from build123d import *

# Parameters (mm, degrees)
F1_DEPTH = 22.5
F2_DEPTH = 25
F3_R     = 5
F5_D     = 22
F5_DEPTH = 6
F5_TIP   = 6.6094668093
F6_D     = 22
F6_DEPTH = 6
F6_TIP   = 6.6094668093
F8_D     = 22
F8_DEPTH = 6
F8_TIP   = 6.6094668093
F9_D     = 22
F9_DEPTH = 6
F9_TIP   = 6.6094668093


with BuildPart() as f1:
    # F0 (on Right) → F1 (new body, symmetric)
    with BuildSketch(Plane.YZ):
        with BuildLine():
            Line((-50, -20), (50, -20))
            Line((50, -20), (37.9778109491, -11.483842507))
            add(Edge.make_bspline(
                [(37.9778109491, -11.483842507), (33.7362140417, -8.5331639275), (28.4293044028, -5.4691263704), (19.5910925664, -4.9491255013), (14.8890013853, -4.8763493822)],
                knots=[0, 0, 0, 0, 0.441705983, 0.8114966727, 0.8114966727, 0.8114966727, 0.8114966727], degree=3))
            Line((14.8890013853, -4.8763493822), (-3.1495152507, 6.404644344))
            Line((-3.1495152507, 6.404644344), (-25.2773519605, 6.404644344))
            Line((-25.2773519605, 6.404644344), (-32.455407083, -4.2915642262))
            Line((-32.455407083, -4.2915642262), (-50, -4.2915642262))
            Line((-50, -4.2915642262), (-50, -20))
        make_face()
    extrude(amount=F1_DEPTH, both=True)

    # F0 (on Right) → F2 (join)
    with BuildSketch(Plane.YZ):
        with BuildLine():
            Line((-50, -20), (50, -20))
            Line((50, -20), (37.9778109491, -11.483842507))
            add(Edge.make_bspline(
                [(37.9778109491, -11.483842507), (33.7362140417, -8.5331639275), (28.4293044028, -5.4691263704), (19.5910925664, -4.9491255013), (14.8890013853, -4.8763493822)],
                knots=[0, 0, 0, 0, 0.441705983, 0.8114966727, 0.8114966727, 0.8114966727, 0.8114966727], degree=3))
            Line((14.8890013853, -4.8763493822), (-3.1495152507, 6.404644344))
            Line((-3.1495152507, 6.404644344), (-25.2773519605, 6.404644344))
            Line((-25.2773519605, 6.404644344), (-32.455407083, -4.2915642262))
            Line((-32.455407083, -4.2915642262), (-50, -4.2915642262))
            Line((-50, -4.2915642262), (-50, -20))
        make_face()
    extrude(amount=F2_DEPTH)

    # F3
    f3_edges = [f1.edges().sort_by_distance(p)[0] for p in [
        (1.25, -25.277352, 6.404644),
        (1.25, -32.455407, -4.291564),
        (1.25, -50, -4.291564),
        (1.25, -3.149515, 6.404644),
        (-11.25, 14.889001, -4.876349),
        (23.75, 14.889001, -4.876349),
        (11.25, 14.889001, -4.876349),
    ]]
    fillet(f3_edges, radius=F3_R)

    # F5
    with Locations(Plane.YZ.offset(25)):
        with Locations((-31.3936918974, -20)):
            Hole(F5_D / 2, depth=F5_DEPTH)
            with Locations((0, 0, -(F5_DEPTH + F5_TIP / 2))):  # 118° drill point
                Cone(0, F5_D / 2, F5_TIP, mode=Mode.SUBTRACT)

    # F6
    with Locations(Plane.YZ.offset(25)):
        with Locations((19.693158567, -20)):
            Hole(F6_D / 2, depth=F6_DEPTH)
            with Locations((0, 0, -(F6_DEPTH + F6_TIP / 2))):  # 118° drill point
                Cone(0, F6_D / 2, F6_TIP, mode=Mode.SUBTRACT)

    # F8
    with Locations(Plane(origin=(-22.5, 0, 0), x_dir=(0, -1, 0), z_dir=(-1, 0, 0))):
        with Locations((-19.701551646, -20)):
            Hole(F8_D / 2, depth=F8_DEPTH)
            with Locations((0, 0, -(F8_DEPTH + F8_TIP / 2))):  # 118° drill point
                Cone(0, F8_D / 2, F8_TIP, mode=Mode.SUBTRACT)

    # F9
    with Locations(Plane(origin=(-22.5, 0, 0), x_dir=(0, -1, 0), z_dir=(-1, 0, 0))):
        with Locations((31.4156152308, -20)):
            Hole(F9_D / 2, depth=F9_DEPTH)
            with Locations((0, 0, -(F9_DEPTH + F9_TIP / 2))):  # 118° drill point
                Cone(0, F9_D / 2, F9_TIP, mode=Mode.SUBTRACT)


solid = f1.part
Design review of the part built by this model. Coordinates are the model's own, in mm. A direction names the side the tool comes from. Round coordinates to 2 decimals unless told otherwise and drop trailing zeros. Order: outer loops, then holes, each group sorted by start corner. A loop starts at its lowest first (then second) coordinate and runs counter-clockwise, first axis right, second up. Notation, with made-up numbers: M 38.5,17.5 L 77.5,17.5 A15 cw 77.5,27.5 Z; hole C 63,81.25 d3. An arc over 180 degrees is marked long. Answer as CSV lines item,"result". Start each with the question number.
1) For pin 1 Ø4 at (y, z) = (20.5, -5) entering from +X; pin 2 Ø2 at (x, z) = (9, -14) entering from +Y; pin 3 Ø4 at (y, z) = (15, -2.5) entering from +X (3 decimals); pin 4 Ø1.5 at (x, z) = (-15, -6.5) entering from +Y, all flat-tipped, find the tip position at first contact; note any pin that passes through.
2) Tool access review of faces 1 (the face through (1, -40, -4.292)), 2 (the face through (1, -50, -15)), 3 (the face through (22, 19.5, -9)): name each direction out of +Z, -Z, +X, -X, +Y, -Y from which nothing blocks a thin tool from reaching the whole face with its end or side.
3) Add section B-B (y = 0). Give the boundary of the cut face in (x, z).
4) Add section A-A (z = 2). Give the boundary of the cut face in (x, y), then the cut area to 3 significant figures.
5) Wall thickness on line 1 along Y through (x, z) = (-13, -16.75); line 2 along Y through (x, z) = (17, -17); line 3 along Z through (x, y) = (-1.5, -35): over which ranges is each line inside the solid? List them lowest first. Write a range as [from, to].
6) The part is to be moulded in two halves that separate along Y. For faces 4 (the face through (1, -1, -20)), 5 (the face through (-19.458, -31.174, -9.003)), 6 (the face through (0.92, 44.07, -15.8)), say which applies: +Y half, -Y half, draft (parallel to the pull), parting line (faces both ways), or undercut.
Resolved:
1,pin 1,"x = 25"
1,pin 2,"y = 42.94"
1,pin 3,"through"
1,pin 4,"y = 30.85"
2,face 1,"+Z, +X, -X, -Y"
2,face 2,"+Z, -Z, +X, -X, -Y"
2,face 3,"-Z, +X"
3,outline,"M -22.5,-20 L 25,-20 L 25,4.43 L -22.5,4.43 Z"
4,outline,"M -22.5,-28.23 L 25,-28.23 L 25,3.89 L -22.5,3.89 Z"
4,area,"1,530 mm^2"
5,line 1,"[-50, -35.44], [-27.39, 15.67], [23.73, 45.41]"
5,line 2,"[-50, -38.45], [-24.33, 12.63], [26.75, 45.76]"
5,line 3,"[-20, -4.29]"
6,face 4,"draft"
6,face 5,"undercut"
6,face 6,"+Y half"
